Input: dimensioned drawing with shaded views. Units: mm. Origin: part minimum x, y, z. Round coordinates to 2 decimals unless told otherwise and drop trailing zeros. Loops run counter-clockwise (first coordinate to the right, second up) from the corner with the lowest first, then second, coordinate; pieces in that order, holes last. Notation, with made-up numbers: (79.25, 72.25) - (92.25, 72.25) arc R12 ccw to (92.25, 88.25) - close; hole circle Ø1 at (-24, -35). An arc over 180 degrees is marked (long way). Answer as a JSON object with one key per item and string values. Group by question number.
Item 1: First-contact query: pin 1 (3 mm diameter, centred on x = 69.75, y = 6.35, fed in from -Z). Flat tip, straight axial feed; report the tip coordinate or a pass-through.
Item 2: Section B-B (x = 69.75). Return the cut outline in (y, z).
Item 3: Section C-C (y = 6). Count the separate pieces of the cut face and the enclosed holes in it, plus the area to 3 significant figures.
Item 4: Draft query along X for the marked faces 1, 2, 3 and 4. Return one class per face: released by +X, released by -X, zero draft, split by the parting line, or undercut.
Item 5: Section A-A (z = 6.35). Return the cut outline in (x, y), plus the area to 3 significant figures.
Item 6: Line query: line 1 (Y direction, x = 15.25, z = 3.5); line 2 (X direction, y = 4.75, z = 6.35); line 3 (X direction, y = 5.75, z = 4). Output: solid intervals per line, ascending.
Item 7: Section D-D (y = 9). Return the cut outline in (x, z) (3 decimals).
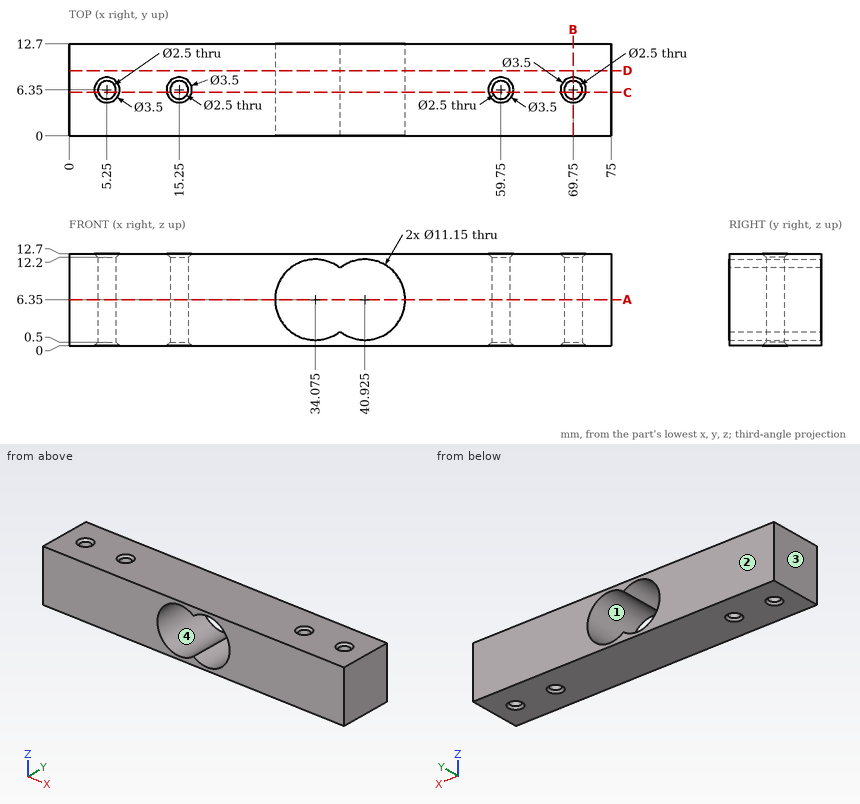
Values:
{
 "1": {"pin 1": "stops at z = 0.25"},
 "2": {"outline": "(0, 0) - (4.6, 0) - (5.1, 0.5) - (5.1, 12.2) - (4.6, 12.7) - (0, 12.7) - close; (7.6, 0.5) - (8.1, 0) - (12.7, 0) - (12.7, 12.7) - (8.1, 12.7) - (7.6, 12.2) - close"},
 "3": {"separate pieces": "5", "enclosed holes": "1", "area": "660 mm^2"},
 "4": {"face 1": "undercut", "face 2": "zero draft", "face 3": "released by -X", "face 4": "undercut"},
 "5": {"outline": "(0, 0) - (28.5, 0) - (28.5, 12.7) - (0, 12.7) - close; (46.5, 0) - (75, 0) - (75, 12.7) - (46.5, 12.7) - close; hole circle Ø2.5 at (5.25, 6.35); hole circle Ø2.5 at (15.25, 6.35); hole circle Ø2.5 at (59.75, 6.35); hole circle Ø2.5 at (69.75, 6.35)", "area": "704 mm^2"},
 "6": {"line 1": "y = 0 to 5.1, 7.6 to 12.7", "line 2": "x = 0 to 28.5, 46.5 to 75", "line 3": "x = 0 to 4.15, 6.35 to 14.15, 16.35 to 29.02, 45.98 to 58.65, 60.85 to 68.65, 70.85 to 75"},
 "7": {"outline": "(0, 0) - (75, 0) - (75, 12.7) - (0, 12.7) - close; hole (37.5, 1.951) arc R5.575 ccw (long way) to (37.5, 10.749) arc R5.575 ccw (long way) to start"}
}
